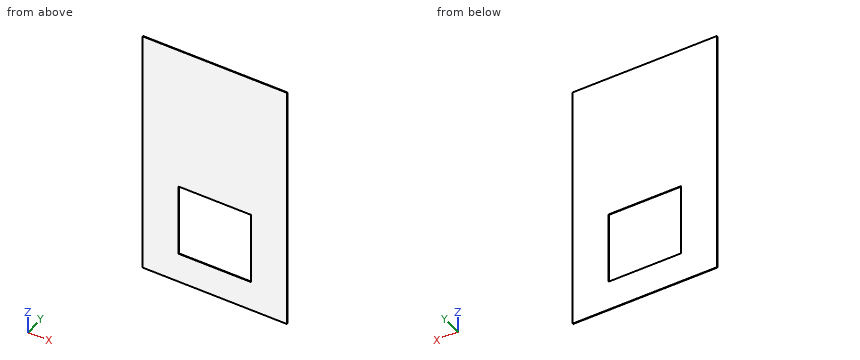
```python
from build123d import *

# Parameters (mm, degrees)
SKETCH1_W               = 1219.2
SKETCH1_H               = 2100.58
BOSS_EXTRUDE1_DEPTH     = 5.55625
SKETCH2_W               = 610.87
SKETCH2_H               = 610.87
CUT_EXTRUDE1_DEPTH      = 1
CUT_EXTRUDE1_DEPTH_BACK = 6.55625


with BuildPart() as part:
    # Sketch1 → Boss-Extrude1 (new body)
    with BuildSketch(Plane(origin=(0, 0, 0), x_dir=(1, 0, 0), z_dir=(0, 1, 0))):
        Rectangle(SKETCH1_W, SKETCH1_H)
    extrude(amount=BOSS_EXTRUDE1_DEPTH)

    # Sketch2 → Cut-Extrude1 (cut, two sides)
    with BuildSketch(Plane(origin=(0, 5.55625, 0), x_dir=(1, 0, 0), z_dir=(0, 1, 0))) as cut_extrude1_sk:
        with Locations((0, 491.49)):
            Rectangle(SKETCH2_W, SKETCH2_H)
    extrude(amount=CUT_EXTRUDE1_DEPTH, mode=Mode.SUBTRACT)
    extrude(cut_extrude1_sk.sketch, amount=-CUT_EXTRUDE1_DEPTH_BACK, mode=Mode.SUBTRACT)


solid = part.part
```
The listing builds one solid part. Answer for the finished solid, in the listing's coordinates (mm). Round coordinates to 2 decimals unless told otherwise and drop trailing zeros. Order: outer loops, then holes, each group sorted by start corner. A loop starts at its lowest first (then second) coordinate and runs counter-clockwise, first axis right, second up. Notation, with made-up numbers: (29, 69) - (86, 69) arc R17 ccw to (86, 102) - close; hole circle Ø3 at (0, -9). An arc over 180 degrees is marked (long way). Put each result on its own line as item: value. Start each with the question number.
(1) Find section B-B (y = 1.85). Give the vertices of the cut face in (x, z) (3 decimals), plus the area to 3 significant figures.
(2) Straight lines are drawn through the part: probe 1 along X at (y, z) = (0.45, -427) (3 decimals); probe 2 along Z at (x, y) = (-132, 0.65) (3 decimals). For each, find the intervals that lie inside material, in ascending order. Write a range as from..to.
(3) Find section A-A (x = -101.5). Give the vertices of the cut face in (y, z) (3 decimals), plus the area to 3 significant figures.
Reply:
1. outline: (-609.6, -1050.29) - (609.6, -1050.29) - (609.6, 1050.29) - (-609.6, 1050.29) - close; hole (-305.435, -796.925) - (305.435, -796.925) - (305.435, -186.055) - (-305.435, -186.055) - close
1. area: 2,190,000 mm^2
2. probe 1: -609.6..-305.435, 305.435..609.6
2. probe 2: -1050.29..-796.925, -186.055..1050.29
3. outline: (0, -1050.29) - (5.556, -1050.29) - (5.556, -796.925) - (0, -796.925) - close; (0, -186.055) - (5.556, -186.055) - (5.556, 1050.29) - (0, 1050.29) - close
3. area: 8,280 mm^2
